Source: CAD feature listing. Evaluate the final solid. Frame: model axes, mm. A direction names the side the tool comes from. Give positions to 0.01 mm unless a question says otherwise; leave off trailing zeros. Order: outer loops, then holes, each group sorted by start corner. A loop starts at its lowest first (then second) coordinate and runs counter-clockwise, first axis right, second up.
```python
from build123d import *

# Parameters (mm, degrees)
ESQUISSE1_R                = 26.506823587
ESQUISSE1_R_2              = 14.875
BOSS_EXTRU_1_DEPTH         = 5
ESQUISSE2_R                = 23.3
ESQUISSE2_R_2              = 15.85
ENL_V_MAT_EXTRU_1_DEPTH    = 2.5
SKETCH1_R                  = 26.506823587
BOSS_EXTRUDE1_DEPTH        = 50
CUT_EXTRUDE6_START         = -46
SKETCH10_R                 = 26.506823587
CUT_EXTRUDE6_DEPTH         = 46
CUT_EXTRUDE7_START         = 23
CUT_EXTRUDE7_DEPTH         = 23
CUT_EXTRUDE8_DEPTH         = 4
SKETCH13_R                 = 14.875
CUT_EXTRUDE9_DEPTH         = 10
TROUS_DE_CENTRAGE_3_0MM1_D = 3


with BuildPart() as part:
    # Esquisse1 → Boss.-Extru.1 (new body)
    with BuildSketch(Plane(origin=(0, 0, 0), x_dir=(1, 0, 0), z_dir=(0, 1, 0))):
        with Locations(Location((0, 0, 0), (0, 0, 270))):
            Circle(ESQUISSE1_R)
        with Locations(Location((0, 0, 0), (0, 0, 270))):
            Circle(ESQUISSE1_R_2, mode=Mode.SUBTRACT)
    extrude(amount=-BOSS_EXTRU_1_DEPTH)

    # Esquisse2 → Enl_v. mat.-Extru.1 (cut)
    with BuildSketch(Plane(origin=(0, 0, 0), x_dir=(1, 0, 0), z_dir=(0, 1, 0))):
        with Locations(Location((0, 0, 0), (0, 0, 270))):
            Circle(ESQUISSE2_R)
        with Locations(Location((0, 0, 0), (0, 0, 270))):
            Circle(ESQUISSE2_R_2, mode=Mode.SUBTRACT)
    extrude(amount=-ENL_V_MAT_EXTRU_1_DEPTH, mode=Mode.SUBTRACT)

    # Sketch1 → Boss-Extrude1 (add)
    with BuildSketch(Plane.XZ.offset(5)):
        with Locations(Location((0, 0, 0), (0, 0, 90))):
            Circle(SKETCH1_R)
    extrude(amount=BOSS_EXTRUDE1_DEPTH)

    # Sketch10 → Cut-Extrude6 (cut)
    with BuildSketch(Plane.XZ.offset(55).offset(CUT_EXTRUDE6_START)):
        with Locations(Location((0, 0, 0), (0, 0, 90))):
            Circle(SKETCH10_R)
    extrude(amount=CUT_EXTRUDE6_DEPTH, mode=Mode.SUBTRACT)

    # Sketch11 → Cut-Extrude7 (cut)
    with BuildSketch(Plane(origin=(0, -2.5, 0), x_dir=(1, 0, 0), z_dir=(0, 1, 0)).offset(CUT_EXTRUDE7_START)):
        with BuildLine():
            Line((-12.221843482, -24.778884374), (-10.256093613, -20.921341826))
            ThreePointArc((-10.256093613, -20.921341826), (-23.070830566, -3.259873772), (-15.651156927, 17.260686164))
            Line((-15.651156927, 17.260686164), (-18.357041818, 20.900818346))
            ThreePointArc((-18.357041818, 20.900818346), (-27.289505672, -3.550750304), (-12.221843482, -24.778884374))
        make_face()
        with BuildLine():
            ThreePointArc((9.561508776, 21.247765763), (21.152163667, 9.771180697), (22.376731607, -6.493988189))
            Line((22.376731607, -6.493988189), (27.230046935, -7.935538889))
            ThreePointArc((27.230046935, -7.935538889), (25.871646158, 11.865956721), (11.723526474, 25.786272467))
            Line((11.723526474, 25.786272467), (9.561508776, 21.247765763))
        make_face()
    extrude(amount=-CUT_EXTRUDE7_DEPTH, mode=Mode.SUBTRACT)

    # Sketch12 → Cut-Extrude8 (cut)
    with BuildSketch(Plane(origin=(0, -2.5, 0), x_dir=(1, 0, 0), z_dir=(0, 1, 0))):
        with BuildLine():
            Line((-17.572262491, 19.845082201), (-13.005635601, 13.70175897))
            ThreePointArc((-13.005635601, 13.70175897), (-18.656508539, -2.969755104), (-8.108525171, -17.062724747))
            Line((-8.108525171, -17.062724747), (-11.712252125, -23.77887396))
            ThreePointArc((-11.712252125, -23.77887396), (-26.270860033, -3.528967239), (-17.572262491, 19.845082201))
        make_face()
        with BuildLine():
            Line((10.940944201, 24.143476068), (7.664960465, 17.26653229))
            ThreePointArc((7.664960465, 17.26653229), (17.123986027, 7.978336844), (18.150504226, -5.238697604))
            Line((18.150504226, -5.238697604), (25.450871211, -7.407081157))
            ThreePointArc((25.450871211, -7.407081157), (24.082160878, 11.075252778), (10.940944201, 24.143476068))
        make_face()
    extrude(amount=-CUT_EXTRUDE8_DEPTH, mode=Mode.SUBTRACT)

    # Sketch13 → Cut-Extrude9 (cut)
    with BuildSketch(Plane(origin=(0, -5, 0), x_dir=(1, 0, 0), z_dir=(0, 1, 0))):
        with Locations(Location((0, 0, 0), (0, 0, 270))):
            Circle(SKETCH13_R)
    extrude(amount=-CUT_EXTRUDE9_DEPTH, mode=Mode.SUBTRACT)

    # Trous de centrage _3.0mm1 (through all)
    with Locations(Plane(origin=(0, -6.5, 0), x_dir=(1, 0, 0), z_dir=(0, 1, 0))):
        with Locations((-21.589234965, -5.972012529), (21.589234965, 5.972012529)):
            Hole(TROUS_DE_CENTRAGE_3_0MM1_D / 2)


solid = part.part
```
1) Reachability of faces 1 (the cylindrical face through (9.161, -1.232, 21.424)), 2 (the cylindrical face through (-18.695, -4.472, 2.716)), 3 (the flat face through (11, -9, 11)), 4 (the flat face through (-9.9, -4.5, 20.4)), 5 (the cylindrical face through (10.152, -5.437, 24.486)) from +Z, -Z, +X, -X, +Y, -Y: full face, straight path, thin tool, end or side. Return the list, or none.
Report:
face 1: +Y
face 2: -X, +Y
face 3: +Z, -Z, +X, -X, -Y
face 4: -X
face 5: +Y, -Y
2) Pin query (flat end, axial travel): pin 1 (5 mm diameter, centred on y = -4.5, z = 1.5, fed in from -X); pin 2 (4 mm diameter, centred on x = -14, z = 17, fed in from +Y); pin 3 (1.5 mm diameter, centred on y = -5, z = 16.5, fed in from -X). Return the tip coordinate at first contact, or that it passes through.
Report:
pin 1: stops at x = -26.51
pin 2: stops at y = -6.5
pin 3: stops at x = -10.43
3) Material intervals for L1, parallel to X at y = -1.75, z = 10.5; L2, parallel to Z at x = 8, y = -0.75; L3, parallel to Z at x = -13, y = -0.75, sorted ascending.
Report:
L1: x = -11.87 to -10.54, 10.54 to 11.87, 20.8 to 24.34
L2: z = -25.27 to -21.88, -13.68 to -12.54, 12.54 to 13.68, 21.88 to 25.27
L3: z = -23.1 to -19.34, -9.07 to -7.23, 7.23 to 9.07
4) Section query A-A, the plane z = 0. Return the cut outline in (x, y) (3 decimals), and give its area (3 significant figures).
Report:
outline: (-26.507, -9) - (-14.875, -9) - (-14.875, 0) - (-15.85, 0) - (-15.85, -2.5) - (-18.891, -2.5) - (-18.891, -6.5) - (-26.507, -6.5) - close; (14.875, -9) - (26.507, -9) - (26.507, -6.5) - (18.891, -6.5) - (18.891, -2.5) - (15.85, -2.5) - (15.85, 0) - (14.875, 0) - close
area: 95.2 mm2
5) Draft query along X for faces 6 (the cylindrical face through (17.043, -4.472, -8.15)), 7 (the cylindrical face through (14.748, -4.437, -1.936)), 8 (the flat face through (-10.994, -1.233, 22.37)), 9 (the flat face through (-3, 0, -24)). Return one class per face: +X half, -X half, draft (parallel to the pull), parting line (faces both ways), or undercut.
Report:
face 6: +X half
face 7: undercut
face 8: -X half
face 9: draft
6) Section query D-D, the plane x = 17.5. Return the cut outline in (y, z), and give its area (3 significant figures).
Report:
outline: (-9, -19.91) - (-6.5, -19.91) - (-6.5, -7.12) - (-2.5, -7.12) - (-2.5, 15.38) - (0, 15.38) - (0, 19.91) - (-9, 19.91) - close
area: 219 mm2
7) Section query B-B, the plane x = 0. Return the cut outline in (y, z) (3 decimals), and give its area (3 significant figures).
Report:
outline: (-9, -26.507) - (0, -26.507) - (0, -23.3) - (-2.5, -23.3) - (-2.5, -15.85) - (0, -15.85) - (0, -14.875) - (-9, -14.875) - close; (-9, 14.875) - (0, 14.875) - (0, 15.85) - (-2.5, 15.85) - (-2.5, 23.3) - (0, 23.3) - (0, 26.507) - (-9, 26.507) - close
area: 172 mm2
